Build history of the part. All positions in model axes, mm. A direction names the side the tool comes from. Round coordinates to 2 decimals unless told otherwise and drop trailing zeros. Loops run counter-clockwise (first coordinate to the right, second up) from the corner with the lowest first, then second, coordinate; pieces in that order, holes last.
from build123d import *

# Parameters (mm, degrees)
F0_R      = 17.5
F1_DEPTH  = 25
F3_R      = 14.5
F4_DEPTH  = 20.5
F1_FACE_R = 17.5
F4_FACE_R = 14.5
F7_D      = 25
F9_D      = 26.6
F9_DEPTH  = 25
F9_TIP    = 7.9914462331


with BuildPart() as f1:
    # F0 (on Top) → F1 (new body)
    with BuildSketch(Plane.XY):
        Circle(F0_R)
    extrude(amount=F1_DEPTH)



with BuildPart() as f4:
    # F3 (on offset) → F4 (new body)
    with BuildSketch(Plane.XY.offset(29.5)):
        Circle(F3_R)
    extrude(amount=F4_DEPTH)


with BuildPart() as f1_1:
    add(f1.part)

    add(f4.part)  # F5 merges F4
    # F1_face (on face) → F5 section 0
    with BuildSketch(Plane.XY.offset(25)):
        Circle(F1_FACE_R)
    # F4_face (on face) → F5 section 1
    with BuildSketch(Plane(origin=(0, 0, 29.5), x_dir=(1, 0, 0), z_dir=(0, 0, -1))):
        Circle(F4_FACE_R)
    loft()

    # F7 (through all)
    with Locations(Plane.XY.offset(50)):
        with Locations((0, 0)):
            Hole(F7_D / 2)

    # F9
    with Locations(Plane(origin=(0, 0, 0), x_dir=(1, 0, 0), z_dir=(0, 0, -1))):
        with Locations((0, 0)):
            Hole(F9_D / 2, depth=F9_DEPTH)
            with Locations((0, 0, -(F9_DEPTH + F9_TIP / 2))):  # 118° drill point
                Cone(0, F9_D / 2, F9_TIP, mode=Mode.SUBTRACT)


solid = f1_1.part
(1) Slice it at C-C on z = 4.5. List the corners of the cut face in (x, y).
Responses:
outline: circle Ø35 at (0, 0); hole circle Ø26.6 at (0, 0)
(2) Slice it at B-B on z = 31.5. List the corners of the cut face in (x, y), plus the area to 3 significant figures.
Responses:
outline: circle Ø29 at (0, 0); hole circle Ø25 at (0, 0)
area: 170 mm2
(3) Which spindle directions (+Z, -Z, +X, -X, +Y, -Y) get a long thin tool onto all of the face, cutting with end or side? Do faces 1 (the face through (6.691, -12.864, 39.606)), 2 (the face through (-13.887, -10.648, 12.325)). Say none if no direction does.
Responses:
face 1: +Z
face 2: +Z, -Z
(4) Pull direction X, two halves, no side cores. Call faces 3 (the face through (-3.17, -14.3, 29.28)), 4 (the face through (12, 7, 0)), 5 (the face through (-6.14, 11.8, 12.67)), 6 (the face through (-11.923, 3.755, 37.569)): +X half, -X half, draft (parallel to the pull), parting line (faces both ways), or undercut.
Responses:
face 3: parting line
face 4: draft
face 5: undercut
face 6: undercut
(5) Slice it at A-A on x = 0. List the corners of the cut face in (y, z), plus the area to 3 significant figures.
Responses:
outline: (-17.5, 0) - (-13.3, 0) - (-13.3, 25) - (-12.5, 25.48) - (-12.5, 50) - (-14.5, 50) - (-14.5, 29.5) - (-17.5, 25) - close; (12.5, 25.48) - (13.3, 25) - (13.3, 0) - (17.5, 0) - (17.5, 25) - (14.5, 29.5) - (14.5, 50) - (12.5, 50) - close
area: 323 mm2
(6) Probe line 1 (Y direction, x = -0.5, z = 14.5); line 2 (Y direction, x = 0, z = 33.5); line 3 (X direction, y = 9.5, z = 37). List the from-to ranges inside material, lowest first.
Responses:
line 1: y = -17.49 to -13.29, 13.29 to 17.49
line 2: y = -14.5 to -12.5, 12.5 to 14.5
line 3: x = -10.95 to -8.12, 8.12 to 10.95
(7) Pin check, flat tips, straight feed: P1, Ø6, axis at x = -2.5, z = 27.5, coming from the -Y side; P2, Ø1, axis at x = 13.5, z = 39, coming from the +Y side; P3, Ø3, axis at y = -11, z = 35, coming from the -X side. Stop position of each tip, or through.
Responses:
P1: stops at y = -17.48
P2: stops at y = 6.42
P3: stops at x = -10.95
